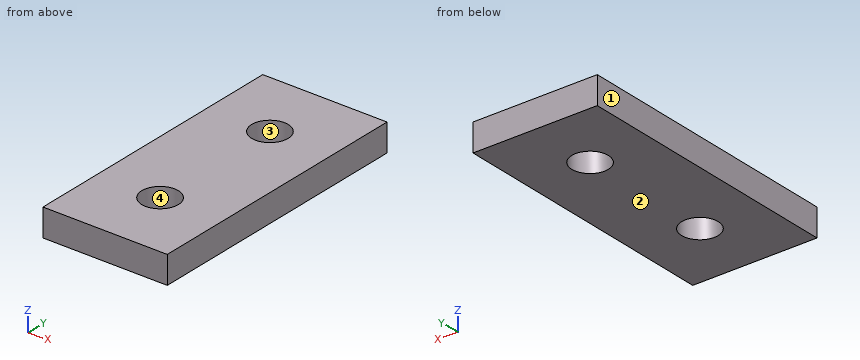
Autodesk Inventor part; units mm, degrees
ref_plane "YZ Plane" through (0, 0, 0) normal (1, 0, 0) x (0, 1, 0)
ref_plane "XZ Plane" through (0, 0, 0) normal (0, 1, 0) x (-1, 0, 0)
ref_plane "XY Plane" through (0, 0, 0) normal (0, 0, 1) x (1, 0, 0)
sketch "Sketch1" plane through (0, 0, 0) normal (0, 0, 1) x (1, 0, 0)
  line L0 (-9, 20) -> (9, 20)
  line L1 (9, 20) -> (9, -20)
  line L2 (9, -20) -> (-9, -20)
  line L3 (-9, -20) -> (-9, 20)
  line L4 (-9, 20) -> (9, -20) construction
  line L5 (9, 20) -> (-9, -20) construction
  circle A0 centre (0, 10) radius 2.65
  line L6 (-9, 0) -> (9, 0) construction
  circle A1 centre (0, -10) radius 2.65
  point P0 (0, 0)
  dimension "d0" = 18
  dimension "d2" = 40
  dimension "d3" = 5.3
  dimension "d4" = 10
  dimension "d5" = 9
extrude "Extrusion1" add sketch "Sketch1" along normal blind 4
properties part number "2 Hole Joining Strip Plate"
Build history of the part. All positions in model axes, mm. Face numbers are marked on the shaded views. Coordinates: 2 decimals unless noted, no trailing zeros. Order: outer loops, then holes, each group sorted by start corner. A loop starts at its lowest first (then second) coordinate and runs counter-clockwise, first axis right, second up. Notation, with made-up numbers: (-20.75, 72) - (16.25, 72) arc R18 ccw to (16.25, 99) - close; hole circle Ø10 at (60, -38.5). An arc over 180 degrees is marked (long way). Write item = value, one per line. Start each with the question number.
1) Saw through at A-A on y = 10. Write the cut outline in (x, z), then the cut area to 3 significant figures.
2) Two-plate mould, pull along X, no slides. Class the marked faces 1, 2, 3 and 4: pulls with the +X half, pulls with the -X half, needs draft (parallel to the pull), parting line crosses it, or undercut.
3) Saw through at D-D on y = -11. Write the cut outline in (x, z), then the cut area to 3 significant figures.
4) Saw through at B-B on x = 0. Write the cut outline in (y, z), then the cut area to 3 significant figures.
5) Saw through at C-C on z = 0.6. Write the cut outline in (x, y).
6) Wall check: line 1 along Y through (x, z) = (0, 2.15); line 2 along Y through (x, z) = (-0.75, 1.9); line 3 along X through (y, z) = (9.5, 1.1). Give the ranges that are in metal, low to high. Write a range as from..to.
From the geometry:
q1.outline = (-9, 0) - (-2.65, 0) - (-2.65, 4) - (-9, 4) - close; (2.65, 0) - (9, 0) - (9, 4) - (2.65, 4) - close
q1.area = 50.8 mm^2
q2.face_1 = pulls with the -X half
q2.face_2 = needs draft
q2.face_3 = undercut
q2.face_4 = undercut
q3.outline = (-9, 0) - (-2.45, 0) - (-2.45, 4) - (-9, 4) - close; (2.45, 0) - (9, 0) - (9, 4) - (2.45, 4) - close
q3.area = 52.4 mm^2
q4.outline = (-20, 0) - (-12.65, 0) - (-12.65, 4) - (-20, 4) - close; (-7.35, 0) - (7.35, 0) - (7.35, 4) - (-7.35, 4) - close; (12.65, 0) - (20, 0) - (20, 4) - (12.65, 4) - close
q4.area = 118 mm^2
q5.outline = (-9, -20) - (9, -20) - (9, 20) - (-9, 20) - close; hole circle Ø5.3 at (0, -10); hole circle Ø5.3 at (0, 10)
q6.line_1 = -20..-12.65, -7.35..7.35, 12.65..20
q6.line_2 = -20..-12.54, -7.46..7.46, 12.54..20
q6.line_3 = -9..-2.6, 2.6..9
